from build123d import *

# Parameters (mm, degrees)
P_IDAT_VYSUNUT_M10_DEPTH   = 120
P_IDAT_VYSUNUT_M10_2_DEPTH = 120
SKICA8_3_W                 = 50
SKICA8_3_H                 = 13
P_IDAT_VYSUNUT_M11_DEPTH   = 5
SKICA12_W                  = 50
SKICA12_H                  = 13
P_IDAT_VYSUNUT_M13_DEPTH   = 5
SKICA13_W                  = 126.2
SKICA13_H                  = 46.2
SKICA13_W_2                = 123.8
SKICA13_H_2                = 43.8
ODEBRAT_VYSUNUT_M1_DEPTH   = 7
ZAOBLIT2_R                 = 2


with BuildPart() as part:
    # Skica8 → P_idat vysunut_m10 (new body)
    with BuildSketch(Plane(origin=(0, 0, 0), x_dir=(0, 0, -1), z_dir=(1, 0, 0))):
        Polygon((6, -3.927822333), (5.008609938, 6.5), (-25, 6.5), (-25, -6.5), (7.5, -6.5), (7.5, -3.785214889), align=None)
    extrude(amount=P_IDAT_VYSUNUT_M10_DEPTH)



with BuildPart() as body_2:
    # Skica8 → P_idat vysunut_m10 2 (new body)
    with BuildSketch(Plane(origin=(0, 0, 0), x_dir=(0, 0, -1), z_dir=(1, 0, 0))):
        Polygon((25, 6.5), (11.035664785, 6.5), (11.973066599, -3.359953158), (10.5, -3.5), (10.5, -6.5), (25, -6.5), align=None)
    extrude(amount=P_IDAT_VYSUNUT_M10_2_DEPTH)


with BuildPart() as part_1:
    add(part.part)

    add(body_2.part)  # P_idat vysunut_m11 merges body 2
    # Skica8_3 → P_idat vysunut_m11 (add)
    with BuildSketch(Plane(origin=(0, 0, 0), x_dir=(0, 0, -1), z_dir=(1, 0, 0))):
        Rectangle(SKICA8_3_W, SKICA8_3_H)
        Polygon((7.5, -6.5), (10.5, -6.5), (10.5, -3.5), (7.5, -3.785214889), align=None)
    extrude(amount=-P_IDAT_VYSUNUT_M11_DEPTH)

    # Skica12 → P_idat vysunut_m13 (add)
    with BuildSketch(Plane(origin=(120, 0, 0), x_dir=(0, 0, -1), z_dir=(1, 0, 0))):
        Rectangle(SKICA12_W, SKICA12_H)
    extrude(amount=P_IDAT_VYSUNUT_M13_DEPTH)

    # Skica13 → Odebrat vysunut_m1 (cut)
    with BuildSketch(Plane.XZ.offset(6.5)):
        with Locations((60, 0)):
            Rectangle(SKICA13_W, SKICA13_H)
        with Locations((60, 0)):
            Rectangle(SKICA13_W_2, SKICA13_H_2, mode=Mode.SUBTRACT)
    extrude(amount=-ODEBRAT_VYSUNUT_M1_DEPTH, mode=Mode.SUBTRACT)

    # Zaoblit2
    zaoblit2_edges = [part_1.edges().sort_by_distance(p)[0] for p in [
        (60, 6.5, -25),
        (-5, 0, 25),
        (60, 6.5, 25),
        (-5, 0, -25),
        (-5, 6.5, 0),
        (125, 0, -25),
        (125, 6.5, 0),
        (125, 0, 25),
    ]]
    fillet(zaoblit2_edges, radius=ZAOBLIT2_R)


solid = part_1.part
Part model, mm, in its own coordinate system. A direction names the side the tool comes from. Coordinates: 2 decimals unless noted, no trailing zeros. Order: outer loops, then holes, each group sorted by start corner. A loop starts at its lowest first (then second) coordinate and runs counter-clockwise, first axis right, second up. Notation, with made-up numbers: M -0.5,-20.5 L 50.5,-20.5 A19 ccw 50.5,14.5 Z; hole C 74.25,9.25 d7. An arc over 180 degrees is marked long. Use a Markdown table: item, result.
(1) Pull direction X, two halves, no side cores. Call faces 1 (the flat face through (59, -1, -25)), 2 (the flat face through (125, -1, 0)), 3 (the flat face through (123.1, -3, 0)), 4 (the flat face through (-3.1, -3, 0)): released by +X, released by -X, zero draft, split by the parting line, or undercut.
A:
| item | result |
|---|---|
| face 1 | zero draft |
| face 2 | released by +X |
| face 3 | undercut |
| face 4 | undercut |
(2) Probe L1, parallel to Z at x = 103.5, y = -5.75; L2, parallel to X at y = -2.25, z = 18.5; L3, parallel to X at y = -1, z = -6.5. List the from-to ranges inside material, lowest first.
A:
| item | result |
|---|---|
| L1 | z = -25 to -23.1, -21.9 to -10.5, -7.5 to 21.9, 23.1 to 25 |
| L2 | x = -5 to -3.1, -1.9 to 121.9, 123.1 to 125 |
| L3 | x = -5 to -3.1, -1.9 to 0, 120 to 121.9, 123.1 to 125 |
(3) Cut at B-B on y = -1.5. Write the cut outline in (x, z), then the cut area to 3 significant figures.
A:
| item | result |
|---|---|
| outline | M -5,-23 A2 ccw -3,-25 L 123,-25 A2 ccw 125,-23 L 125,23 A2 ccw 123,25 L -3,25 A2 ccw -5,23 Z; M -1.9,-21.9 L 121.9,-21.9 L 121.9,21.9 L -1.9,21.9 Z; hole M -3.1,-23.1 L 123.1,-23.1 L 123.1,23.1 L -3.1,23.1 Z; hole M 0,-11.8 L 120,-11.8 L 120,-5.77 L 0,-5.77 Z |
| area | 5,370 mm^2 |
(4) Tool access for faces 5 (the flat face through (59, -1, 25)), 6 (the flat face through (59.2, 1.6, -11.5)), 7 (the flat face through (121.9, -3, 0)), 8 (the flat face through (59, -5, -7.5)), 9 (the flat face through (59.16, 1.21, -5.51)): list every direction of +Z, -Z, +X, -X, +Y, -Y with a clear straight run to the whole face (end or side of a thin tool).
A:
| item | result |
|---|---|
| face 5 | +Z, +X, -X, +Y, -Y |
| face 6 | none |
| face 7 | -Y |
| face 8 | +Y, -Y |
| face 9 | +Y |
(5) Cut at A-A on x = 46. Write the cut outline in (y, z), then the cut area to 3 significant figures.
A:
| item | result |
|---|---|
| outline | M -6.5,-25 L 4.5,-25 A2 ccw 6.5,-23 L 6.5,-11.04 L -3.36,-11.97 L -3.5,-10.5 L -6.5,-10.5 L -6.5,-21.9 L 0.5,-21.9 L 0.5,-23.1 L -6.5,-23.1 Z; M -6.5,-7.5 L -3.79,-7.5 L -3.93,-6 L 6.5,-5.01 L 6.5,23 A2 ccw 4.5,25 L -6.5,25 L -6.5,23.1 L 0.5,23.1 L 0.5,21.9 L -6.5,21.9 Z |
| area | 562 mm^2 |
